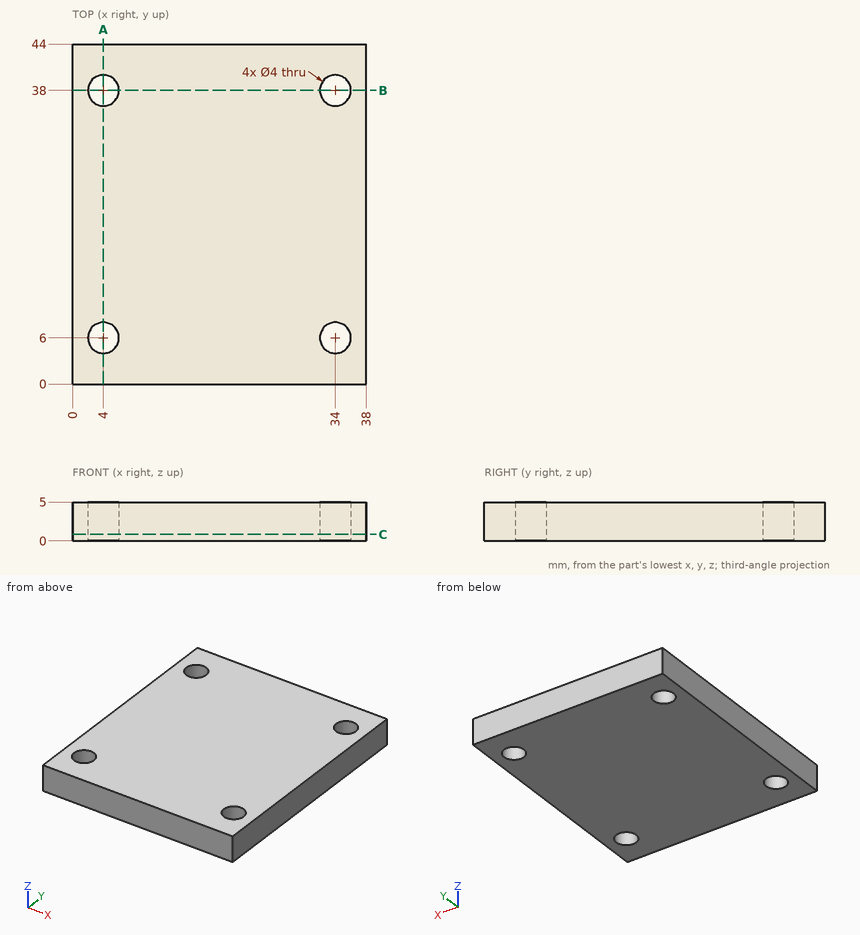
Design review of the part shown in the three views and the two pictorial views. Dimensions are in mm from the part's minimum x, y and z. Round coordinates to 2 decimals unless told otherwise and drop trailing zeros. Loops run counter-clockwise (first coordinate to the right, second up) from the corner with the lowest first, then second, coordinate; pieces in that order, holes last.
Q1. Insertion check: pin 1 Ø3 at (x, y) = (34, 6) entering from +Z. The pin has a flat end and moves straight along its axis. Give the tip position at first contact, or say it passes through.
Result sheet:
pin 1: passes through
Q2. Add section A-A on x = 4. Write out the cut boundary in (y, z), plus the area to 3 significant figures.
Result sheet:
outline: (0, 0) - (4, 0) - (4, 5) - (0, 5) - close; (8, 0) - (36, 0) - (36, 5) - (8, 5) - close; (40, 0) - (44, 0) - (44, 5) - (40, 5) - close
area: 180 mm2
Q3. To check wall thickness, follow line 1 along Y through (x, z) = (34, 2.6); line 2 along X through (y, z) = (39, 3.15); line 3 along Y through (x, z) = (35.5, 4.7). State the ranges of each line that lie inside material, in increasing order.
Result sheet:
line 1: y = 0 to 4, 8 to 36, 40 to 44
line 2: x = 0 to 2.27, 5.73 to 32.27, 35.73 to 38
line 3: y = 0 to 4.68, 7.32 to 36.68, 39.32 to 44
Q4. Add section C-C on z = 0.85. Write out the cut boundary in (x, y).
Result sheet:
outline: (0, 0) - (38, 0) - (38, 44) - (0, 44) - close; hole circle Ø4 at (4, 6); hole circle Ø4 at (4, 38); hole circle Ø4 at (34, 6); hole circle Ø4 at (34, 38)
Q5. Add section B-B on y = 38. Write out the cut boundary in (x, z), plus the area to 3 significant figures.
Result sheet:
outline: (0, 0) - (2, 0) - (2, 5) - (0, 5) - close; (6, 0) - (32, 0) - (32, 5) - (6, 5) - close; (36, 0) - (38, 0) - (38, 5) - (36, 5) - close
area: 150 mm2
